Work out the finished part from the listing and answer in its coordinate system (mm). Round coordinates to 2 decimals unless told otherwise and drop trailing zeros. Order: outer loops, then holes, each group sorted by start corner. A loop starts at its lowest first (then second) coordinate and runs counter-clockwise, first axis right, second up. Notation, with made-up numbers: (34, 80.25) - (70, 80.25) arc R17 ccw to (70, 112.25) - close; hole circle Ø7 at (-17, 37.5). An arc over 180 degrees is marked (long way). One line per question, with ' | ' between items. Start each with the question number.
from build123d import *

# Parameters (mm, degrees)
IZIM1_W                     = 390
IZIM1_H                     = 20
IZIM1_R                     = 2
Y_KSEKLIK_EKSTR_ZYON1_DEPTH = 3
IZIM2_W                     = 40
IZIM2_H                     = 50
Y_KSEKLIK_EKSTR_ZYON2_DEPTH = 3


with BuildPart() as part:
    # Çizim1 → Yükseklik-Ekstrüzyon1 (new body)
    with BuildSketch(Plane(origin=(0, 0, 0), x_dir=(0, 0, -1), z_dir=(1, 0, 0))):
        with Locations((195, 10)):
            Rectangle(IZIM1_W, IZIM1_H)
        with Locations((10, 10)):
            Circle(IZIM1_R, mode=Mode.SUBTRACT)
        with Locations((84, 10)):
            Circle(IZIM1_R, mode=Mode.SUBTRACT)
        with Locations((158, 10)):
            Circle(IZIM1_R, mode=Mode.SUBTRACT)
        with Locations((232, 10)):
            Circle(IZIM1_R, mode=Mode.SUBTRACT)
        with Locations((306, 10)):
            Circle(IZIM1_R, mode=Mode.SUBTRACT)
        with Locations((380, 10)):
            Circle(IZIM1_R, mode=Mode.SUBTRACT)
    extrude(amount=Y_KSEKLIK_EKSTR_ZYON1_DEPTH)

    # Çizim2 → Yükseklik-Ekstrüzyon2 (add)
    with BuildSketch(Plane(origin=(3, 0, 0), x_dir=(0, 0, -1), z_dir=(1, 0, 0))):
        with Locations((195, 45)):
            Rectangle(IZIM2_W, IZIM2_H)
        with BuildLine():
            Line((197, 64), (197, 24))
            ThreePointArc((197, 24), (195, 22), (193, 24))
            Line((193, 24), (193, 64))
            ThreePointArc((193, 64), (195, 66), (197, 64))
        make_face(mode=Mode.SUBTRACT)
    extrude(amount=-Y_KSEKLIK_EKSTR_ZYON2_DEPTH)


solid = part.part
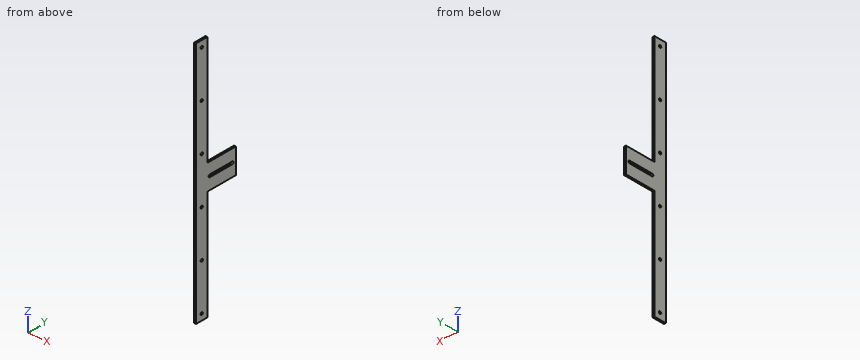
1) Section B-B on x = 2.2 is taken. Give the vertices of the cut face in (y, z), and give its area (3 significant figures).
2) Flat-ended cylindrical pins translate along their axes: pin 1 (0.9 mm diameter, centred on x = 1, y = 40.5, fed in from +Z); pin 2 (0.9 mm diameter, centred on x = 1.5, y = 53, fed in from -Z). Find the tip coordinate at first contact, or state that the pin passes through.
3) Straight lines are drawn through the part: line 1 (Y direction, x = 1.15, z = -232); line 2 (Z direction, x = 1.35, y = 42); line 3 (Z direction, x = 0.7, y = 20.5). For each, find the intervals that lie inside material, in ascending order.
4) Section C-C on z = -89.5 is taken. Give the vertices of the cut face in (x, y).
5) Section A-A on y = 39 is taken. Give the vertices of the cut face in (x, z), and give its area (3 significant figures).
Recorded:
1) outline: (0, -390) - (20, -390) - (20, -215) - (70, -215) - (70, -175) - (20, -175) - (20, 0) - (0, 0) - close; hole circle Ø4 at (10, -380); hole circle Ø4 at (10, -306); hole circle Ø4 at (10, -232); hole circle Ø4 at (10, -158); hole circle Ø4 at (10, -84); hole circle Ø4 at (10, -10); hole (24, -197) - (64, -197) arc R2 ccw to (64, -193) - (24, -193) arc R2 ccw to start | area: 9,550 mm²
2) pin 1: stops at z = -175 | pin 2: stops at z = -215
3) line 1: y = 0 to 8, 12 to 20 | line 2: z = -215 to -197, -193 to -175 | line 3: z = -215 to -175
4) outline: (0, 0) - (3, 0) - (3, 20) - (0, 20) - close
5) outline: (0, -215) - (3, -215) - (3, -197) - (0, -197) - close; (0, -193) - (3, -193) - (3, -175) - (0, -175) - close | area: 108 mm²
